Check sheet for the modelled part. Datum: model origin and axes. Units: mm. Face numbers are marked on the shaded views. A direction names the side the tool comes from. Coordinates: 2 decimals unless noted, no trailing zeros. Write each loop counter-clockwise with the first axis right and the second up, starting at its lowest first coordinate (ties: lowest second). Pieces come first, ordered by that corner, then holes. Notation, with made-up numbers: M 83.25,64.25 L 131.25,64.25 A23 ccw 131.25,78.25 Z; hole C -31,-8 d2. An arc over 180 degrees is marked long. Answer as CSV lines item,"result". Start each with the question number.
1) Section check B-B (x = 0). Record the cut outline in (y, z).
2) Access from +Z, -Z, +X, -X, +Y, -Y to the whole of each face (thin tool, end or side, straight path). Record for the marked faces 4 and 5.
3) Draft check along Z on the marked faces 1, 2 and 3. Enter one of: +Z half, -Z half, draft (parallel to the pull), parting line (faces both ways), or undercut.
4) Go/stop test with flat-tipped pins: pin 1 Ø4 at (x, y) = (-2, 8) entering from +Z; pin 2 Ø1.5 at (y, z) = (6, -1.5) entering from -X; pin 3 Ø6 at (x, z) = (8.5, -5.5) entering from +Y; pin 4 Ø1.5 at (x, y) = (1, 2.5) entering from -Z. Record where each tip stops, or that it passes through.
5) Material ranges on L1, parallel to X at y = 1.9, z = 0; L2, parallel to Y at x = 9, z = 9; L3, parallel to Z at x = -2.5, y = 7.5, recorded low to high. Write a range as [from, to].
6) Section check D-D (z = 4.75). Record the cut outline in (x, y), and give its area (3 significant figures).
7) Section check C-C (y = 1.25). Record the cut outline in (x, z), and give its area (3 significant figures).
8) Section check A-A (z = 0). Record the cut outline in (x, y).
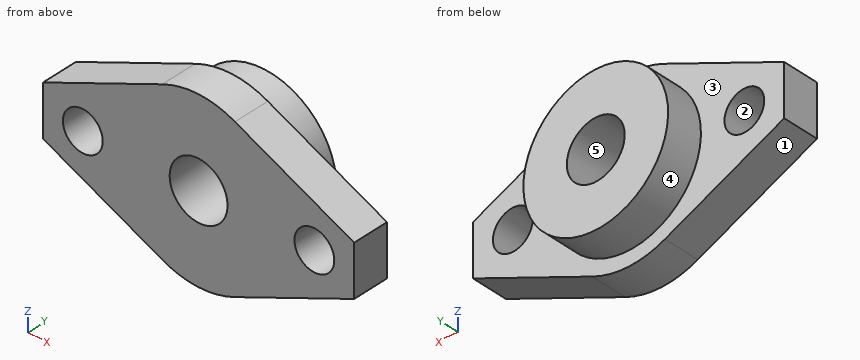
from build123d import *

# Parameters (mm, degrees)
SKETCH1_R           = 2.75
SKETCH1_R_2         = 12
BOSS_EXTRUDE1_DEPTH = 5
SKETCH2_R           = 10
BOSS_EXTRUDE2_DEPTH = 5
CUT_EXTRUDE1_REACH  = 28.575
SKETCH3_R           = 4


with BuildPart() as part:
    # Sketch1 → Boss-Extrude1 (new body)
    # profile 1 of 3: a face of its own
    with BuildSketch(Plane(origin=(0, 0, 0), x_dir=(1, 0, 0), z_dir=(0, 1, 0))):
        with BuildLine():
            Line((21.5, 3.5), (5.025448323, 10.897011937))
            ThreePointArc((5.025448323, 10.897011937), (10.10706139, 6.468949688), (12, 0))
            ThreePointArc((12, 0), (10.10706139, -6.468949688), (5.025448323, -10.897011937))
            Line((5.025448323, -10.897011937), (21.5, -3.5))
            Line((21.5, -3.5), (21.5, 3.5))
        make_face()
        with Locations(Location((16, 0, 0), (0, 0, 270))):
            Circle(SKETCH1_R, mode=Mode.SUBTRACT)
    # profile 2 of 3: a face of its own
    with BuildSketch(Plane(origin=(0, 0, 0), x_dir=(1, 0, 0), z_dir=(0, 1, 0))):
        Circle(SKETCH1_R_2)
    # profile 3 of 3: a face of its own
    with BuildSketch(Plane(origin=(0, 0, 0), x_dir=(1, 0, 0), z_dir=(0, 1, 0))):
        with BuildLine():
            Line((-5.025448323, 10.897011937), (-21.5, 3.5))
            Line((-21.5, 3.5), (-21.5, -3.5))
            Line((-21.5, -3.5), (-5.025448323, -10.897011937))
            ThreePointArc((-5.025448323, -10.897011937), (-12, 0), (-5.025448323, 10.897011937))
        make_face()
        with Locations(Location((-16, 0, 0), (0, 0, 270))):
            Circle(SKETCH1_R, mode=Mode.SUBTRACT)
    extrude(amount=BOSS_EXTRUDE1_DEPTH)

    # Sketch2 → Boss-Extrude2 (add)
    with BuildSketch(Plane(origin=(0, 5, 0), x_dir=(1, 0, 0), z_dir=(0, 1, 0))):
        with Locations(Location((0, 0, 0), (0, 0, 270))):
            Circle(SKETCH2_R)
    extrude(amount=BOSS_EXTRUDE2_DEPTH)

    # Sketch3 → Cut-Extrude1 (cut, up to next)
    with BuildSketch(Plane(origin=(0, 10, 0), x_dir=(1, 0, 0), z_dir=(0, 1, 0)), mode=Mode.PRIVATE) as cut_extrude1_sk1:
        with Locations(Location((0, 0, 0), (0, 0, 270))):
            Circle(SKETCH3_R)
    cut_extrude1_tool1 = extrude(cut_extrude1_sk1.sketch, amount=-CUT_EXTRUDE1_REACH, mode=Mode.PRIVATE) & part.part
    add(cut_extrude1_tool1.solids().sort_by_distance((0, 10, 0))[0], mode=Mode.SUBTRACT)


solid = part.part
Results found:
1,outline,"M 0,-12 L 5,-12 L 5,-10 L 10,-10 L 10,-4 L 0,-4 Z; M 0,4 L 10,4 L 10,10 L 5,10 L 5,12 L 0,12 Z"
2,face 4,"+Y"
2,face 5,"+Y, -Y"
3,face 1,"-Z half"
3,face 2,"undercut"
3,face 3,"draft"
4,pin 1,"stops at z = 10"
4,pin 2,"stops at x = -9.97"
4,pin 3,"stops at y = 10"
4,pin 4,"stops at z = -12"
5,L1,"x = [-21.5, -18.75], [-13.25, -4], [4, 13.25], [18.75, 21.5]"
5,L2,"y = [0, 5]"
5,L3,"z = [-9.68, -3.12], [3.12, 9.68]"
6,outline,"M -18.72,0 L 18.72,0 L 18.72,5 L 8.8,5 L 8.8,10 L -8.8,10 L -8.8,5 L -18.72,5 Z"
6,area,"275 mm2"
7,outline,"M -21.5,-3.5 L -5.03,-10.9 A12 ccw 5.03,-10.9 L 21.5,-3.5 L 21.5,3.5 L 5.03,10.9 A12 ccw -5.03,10.9 L -21.5,3.5 Z; hole C -16,0 d5.5; hole C 0,0 d8; hole C 16,0 d5.5"
7,area,"611 mm2"
8,outline,"M -21.5,0 L -18.75,0 L -18.75,5 L -21.5,5 Z; M -13.25,0 L -4,0 L -4,10 L -10,10 L -10,5 L -13.25,5 Z; M 4,0 L 13.25,0 L 13.25,5 L 10,5 L 10,10 L 4,10 Z; M 18.75,0 L 21.5,0 L 21.5,5 L 18.75,5 Z"
